Geometry check sheet. Reference: the model listing, model coordinates, mm. Coordinates: 2 decimals unless noted, no trailing zeros. Loops run counter-clockwise (first coordinate to the right, second up) from the corner with the lowest first, then second, coordinate; pieces in that order, holes last.
Autodesk Inventor part; units mm, degrees
ref_plane "YZ Plane" through (0, 0, 0) normal (1, 0, 0) x (0, 1, 0)
ref_plane "XZ Plane" through (0, 0, 0) normal (0, 1, 0) x (-1, 0, 0)
ref_plane "XY Plane" through (0, 0, 0) normal (0, 0, 1) x (1, 0, 0)
sketch "Sketch1" plane through (0, 0, 0) normal (0, 0, 1) x (1, 0, 0)
  circle A0 centre (0, 0) radius 13.97
  circle A1 centre (0, 0) radius 10.795
  dimension "d0" = 27.94
  dimension "d2" = 21.59
extrude "Extrusion1" add sketch "Sketch1" along normal blind 13.335
sketch "Sketch2" plane through (0, 0, 13.335) normal (0, 0, 1) x (1, 0, 0)
  circle A0 centre (0, 0) radius 13.97
extrude "Extrusion2" add sketch "Sketch2" along normal blind 3.175
fillet "Fillet1" radius 3.175 1 edges at (-13.97, 0, 16.51)
sketch "Sketch3" plane through (0, 0, 0) normal (0, 0, -1) x (-1, 0, 0)
  circle A0 centre (0, 0) radius 10.795
  circle A1 centre (0, 0) radius 13.97
extrude "Extrusion3" add sketch "Sketch3" along normal blind 1.27
sketch "Sketch4" plane through (0, 0, -1.27) normal (0, 0, -1) x (-1, 0, 0)
  circle A0 centre (0, 0) radius 10.795
  circle A1 centre (0, 0) radius 13.97
extrude "Extrusion4" cut sketch "Sketch4" along normal blind 5.715
sketch "Sketch5" plane through (0, 0, -1.27) normal (0, 0, -1) x (-1, 0, 0)
  circle A0 centre (0, 0) radius 10.795
  circle A1 centre (0, 0) radius 13.97
extrude "Extrusion5" add sketch "Sketch5" along normal blind 8.255
properties part number "Long Cap" material "PVC-Piping"
(1) Sectioned sample at A-A on z = 6.5. Record the cut outline in (x, y) (3 decimals), and give its area (3 significant figures).
Findings:
outline: circle Ø27.94 at (0, 0); hole circle Ø21.59 at (0, 0)
area: 247 mm2
(2) Gauge pin test, flat ends, axial feed: pin 1 Ø10 at (y, z) = (-6.5, 0) entering from -X; pin 2 Ø3 at (x, z) = (-4.5, 1) entering from +Y; pin 3 Ø2 at (y, z) = (3.5, 4) entering from -X. Record the tip position at first contact, or that the pin passes through.
Findings:
pin 1: stops at x = -13.89
pin 2: stops at y = 13.64
pin 3: stops at x = -13.74
(3) Draft check along Y on faces 1 (the flat face through (0, 0, 13.335)), 2 (the flat face through (0, 0, 16.51)). Enter one of: +Y half, -Y half, draft (parallel to the pull), parting line (faces both ways), or undercut.
Findings:
face 1: undercut
face 2: draft
(4) Scan lines: L1, parallel to Y at x = 0, z = -0.7 (3 decimals); L2, parallel to Z at x = 4, y = -5 (3 decimals). Record each from-to range of solid material in increasing order.
Findings:
L1: y = -13.97 to -10.795, 10.795 to 13.97
L2: z = 13.335 to 16.51
(5) Sectioned sample at B-B on x = 0. Record the cut outline in (y, z) (3 decimals), and give its area (3 significant figures).
Findings:
outline: (-13.97, -9.525) - (-10.795, -9.525) - (-10.795, 13.335) - (10.795, 13.335) - (10.795, -9.525) - (13.97, -9.525) - (13.97, 13.335) arc R3.175 ccw to (10.795, 16.51) - (-10.795, 16.51) arc R3.175 ccw to (-13.97, 13.335) - close
area: 230 mm2
